Verification items for the finished model (mm, model axes). A direction names the side the tool comes from. Give positions to 0.01 mm unless a question says otherwise; leave off trailing zeros. Order: outer loops, then holes, each group sorted by start corner. A loop starts at its lowest first (then second) coordinate and runs counter-clockwise, first axis right, second up. Notation, with made-up numbers: (-20.5, 86.25) -> (28.5, 86.25) arc R24 ccw to (28.5, 105.25) -> close; hole circle Ø3 at (86, 49.25). An arc over 180 degrees is marked (long way). Return JSON: item names as keys, results as strings. Group by question number.
(1) Cross-section at A-A on x = 3.75. Enter the section's corners in (y, z).
(2) Cross-section at C-C on x = -6. Enter the section's corners in (y, z).
(3) Release check for a two-part mould opening along Y. For faces 1 (the face through (-9.5, 0, -3)), 2 (the face through (-1.01, 4.91, 1.55)), 3 (the face through (-8.268, -2.155, 1.267)) record: pulls with the +Y half, pulls with the -Y half, needs draft (parallel to the pull), parting line crosses it, or undercut.
(4) Tool access check on faces 4 (the face through (0, 0.1, -3.4)), 5 (the face through (-8, 0, 2.5)). Record the directions out of +Z, -Z, +X, -X, +Y, -Y that give a thin tool (end or side, any length) a straight path to the whole face; none if there is none.
(5) Depth check by flat-ended pin: pin 1 Ø3 at (x, y) = (-8, 0) entering from -Z; pin 2 Ø5 at (x, z) = (-6.5, -0.5) entering from +Y; pin 3 Ø0.6 at (y, z) = (2.5, -0.5) entering from -X; pin 4 Ø1.2 at (x, y) = (-9, 0) entering from +Z. Enter the tip coordinate at first touch or a pass-through.
(6) Thickness scan on line 1 along Z through (x, y) = (-8, -2.5); line 2 along Y through (x, z) = (-7.25, 1); line 3 along X through (y, z) = (-2.5, -0.5). Record the ranges inside material, lowest first.
(7) Cross-section at D-D on z = 4.5. Enter the section's corners in (x, y), then the cut area to 3 significant figures.
(8) Cross-section at B-B on y = 4.75. Enter the section's corners in (x, z).
from build123d import *

# Parameters (mm, degrees)
CUT_EXTRUDE3_DEPTH = 2.5


with BuildPart() as part:
    # Sketch1 → Revolve1 (revolve)
    with BuildSketch(Plane.XY):
        Polygon((-9.5, 0), (8, 0), (8, 3), (0, 3), (0, 5.15), (-2, 5.15), (-2, 4), (-9.5, 4), (-9, 3.2), (-9.5, 3.2), align=None)
    revolve(axis=Axis((-9.190479794, 0, 0), (1, 0, 0)))

    # Sketch5 → Cut-Revolve1 (revolve, cut)
    with BuildSketch(Plane.XY):
        Polygon((-9.5, 2.5), (-7, 2.5), (-5.497848452, 0), (-9.5, 0), align=None)
    revolve(axis=Axis((-9.5, 0, 0), (1, 0, 0)), mode=Mode.SUBTRACT)

    # Sketch4 → Cut-Extrude3 (cut)
    with BuildSketch(Plane(origin=(-9.5, 0, 0), x_dir=(0, 0, -1), z_dir=(1, 0, 0))):
        Polygon((0, 2.886751346), (-2.5, 1.443375673), (-2.5, -1.443375673), (0, -2.886751346), (2.5, -1.443375673), (2.5, 1.443375673), align=None)
    extrude(amount=CUT_EXTRUDE3_DEPTH, mode=Mode.SUBTRACT)


solid = part.part
Verdict:
{
 "1": {"outline": "circle Ø6 at (0, 0)"},
 "2": {"outline": "circle Ø8 at (0, 0); hole circle Ø1.67 at (0, 0)"},
 "3": {"face 1": "needs draft", "face 2": "parting line crosses it", "face 3": "undercut"},
 "4": {"face 4": "+X", "face 5": "-X"},
 "5": {"pin 1": "z = -4", "pin 2": "y = 4", "pin 3": "x = -9.5", "pin 4": "z = 4"},
 "6": {"line 1": "-3.12 to -0.67, 0.67 to 3.12", "line 2": "-3.87 to -2.31, 2.31 to 3.87", "line 3": "-7 to 8"},
 "7": {"outline": "(-2, -2.5) -> (0, -2.5) -> (0, 2.5) -> (-2, 2.5) -> close", "area": "10.0 mm²"},
 "8": {"outline": "(-2, -1.99) -> (0, -1.99) -> (0, 1.99) -> (-2, 1.99) -> close"}
}
